Job drawing, mm, ordinate dimensions from the low corner. One solid piece. A direction names the side the tool comes from. Give positions to 0.01 mm unless a question says otherwise; leave off trailing zeros. Write each loop counter-clockwise with the first axis right and the second up, starting at its lowest first coordinate (ties: lowest second). Pieces come first, ordered by that corner, then holes. Notation, with made-up numbers: (-32, 46.25) - (-25, 46.25) arc R17 ccw to (-25, 53.25) - close; hole circle Ø3 at (-18.75, 25). An arc over 180 degrees is marked (long way). Answer in a Markdown table with one row per item. Add a question column.
1. Which spindle directions (+Z, -Z, +X, -X, +Y, -Y) get a long thin tool onto all of the face, cutting with end or side? Do the marked faces 4, 5 and 6. Say none if no direction does.
2. Band-saw the part on D-D on y = 15.5. State how many separate pieces and enclosed holes the cut face has, plus the area to 3 significant figures.
3. Probe line 1 along X through (y, z) = (10.5, 23); line 2 along Z through (x, y) = (82, 19.25); line 3 along X through (y, z) = (17, 18) (3 decimals). List the from-to ranges inside material, lowest first.
4. Band-saw the part on B-B on z = 10. Write the cut outline in (x, y), plus the area to 3 significant figures.
5. Band-saw the part on A-A on x = 13. Write the cut outline in (y, z), plus the area to 3 significant figures.
6. Drop flat-ended pins along their axis: pin 1 Ø9.5 at (x, z) = (13, 23) entering from -Y; pin 2 Ø5.5 at (x, y) = (66.5, 9.5) entering from -Z; pin 3 Ø6 at (x, z) = (20.5, 39.5) entering from +Y; pin 4 Ø1 at (x, z) = (65.5, 43) entering from -Y. Give the stop position or say it passes through.
7. Pull direction X, two halves, no side cores. Call the marked faces 1, 2 and 3: released by +X, released by -X, zero draft, split by the parting line, or undercut.
8. Band-saw the part on C-C on x = 39.25. Write the cut outline in (y, z), plus the area to 3 significant figures.
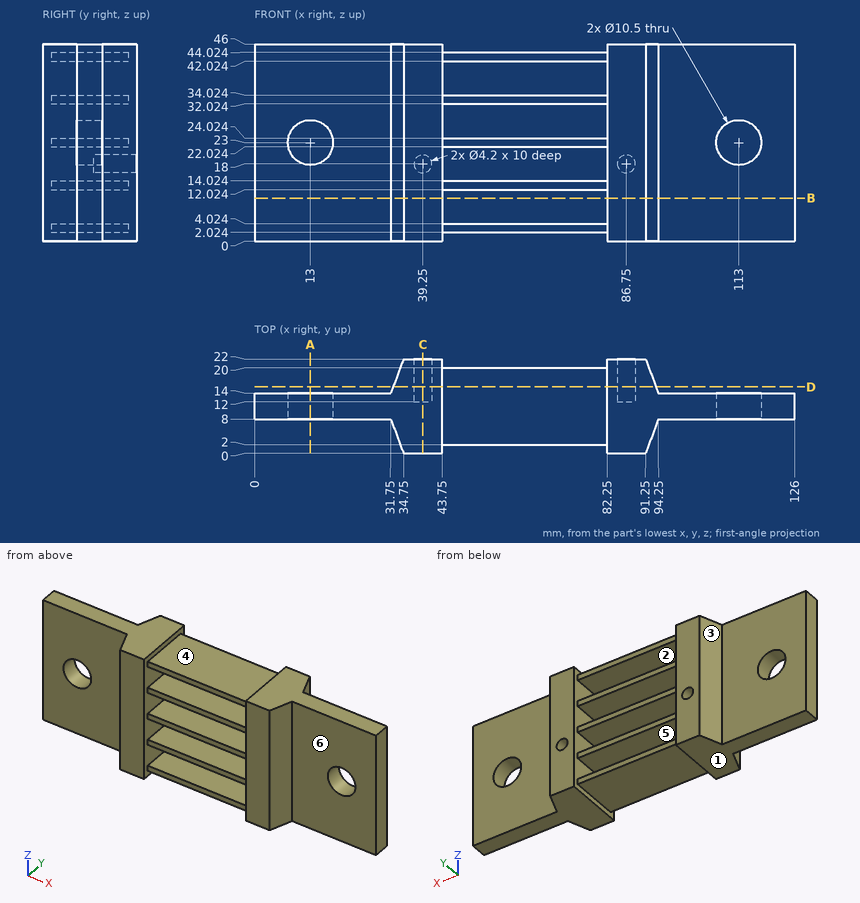
Values:
| question | item | result |
|---|---|---|
| 1 | face 4 | +Z, +Y, -Y |
| 1 | face 5 | +Y, -Y |
| 1 | face 6 | +Z, -Z, +X, -Y |
| 2 | separate pieces | 1 |
| 2 | enclosed holes | 6 |
| 2 | area | 1,410 mm² |
| 3 | line 1 | x = 0 to 7.75, 18.25 to 107.75, 118.25 to 126 |
| 3 | line 2 | z = 2.02 to 4.02, 12.02 to 14.02, 22.02 to 24.02, 32.02 to 34.02, 42.02 to 44.02 |
| 3 | line 3 | x = 32.875 to 37.15, 41.35 to 43.75, 82.25 to 84.65, 88.85 to 93.125 |
| 4 | outline | (0, 8) - (31.75, 8) - (34.75, 0) - (43.75, 0) - (43.75, 22) - (34.75, 22) - (31.75, 14) - (0, 14) - close; (82.25, 0) - (91.25, 0) - (94.25, 8) - (126, 8) - (126, 14) - (94.25, 14) - (91.25, 22) - (82.25, 22) - close |
| 4 | area | 861 mm² |
| 5 | outline | (8, 0) - (14, 0) - (14, 17.75) - (8, 17.75) - close; (8, 28.25) - (14, 28.25) - (14, 46) - (8, 46) - close |
| 5 | area | 213 mm² |
| 6 | pin 1 | passes through |
| 6 | pin 2 | stops at z = 2.02 |
| 6 | pin 3 | stops at y = 14 |
| 6 | pin 4 | stops at y = 2 |
| 7 | face 1 | zero draft |
| 7 | face 2 | undercut |
| 7 | face 3 | released by -X |
| 8 | outline | (0, 0) - (22, 0) - (22, 15.9) - (12, 15.9) - (12, 20.1) - (22, 20.1) - (22, 46) - (0, 46) - close |
| 8 | area | 970 mm² |
